from build123d import *

# Parameters (mm, degrees)
F1_DEPTH = 63.5
F2_DEPTH = 25.4
F0_W     = 25.3307413936
F0_H     = 19.05
F3_DEPTH = 50.8


with BuildPart() as f1:
    # F0 (on Front) → F1 (new body, symmetric)
    with BuildSketch(Plane.XZ):
        Polygon((-41.275, -9.525), (41.275, -9.525), (41.275, 9.525), (22.225, 9.525), (-41.275, 9.525), align=None)
    extrude(amount=F1_DEPTH, both=True)

    # F0 (on Front) → F2 (join, symmetric)
    with BuildSketch(Plane.XZ):
        with BuildLine():
            add(Edge.make_bspline(
                [(-41.275, 9.525), (-41.1319843278, 26.4440384857), (9.9134722481, 58.1405185942), (52.9354553425, 61.6699741315)],
                knots=[0, 0, 0, 0, 107.9558196003, 107.9558196003, 107.9558196003, 107.9558196003], degree=3))
            Line((-41.275, 9.525), (22.225, 9.525))
            Line((22.225, 9.525), (22.225, 27.0002))
            ThreePointArc((22.225, 27.0002), (31.0066586187, 50.1579487338), (52.9354553425, 61.6699741315))
        make_face()
    extrude(amount=F2_DEPTH, both=True)

    # F0 (on Front) → F3 (join, symmetric)
    with BuildSketch(Plane.XZ):
        with BuildLine():
            Line((22.225, 9.525), (41.275, 9.525))
            Line((41.275, 9.525), (41.275, 27.0002))
            ThreePointArc((41.275, 27.0002), (45.9246798487, 38.2255201513), (57.15, 42.8752))
            Line((57.15, 42.8752), (60.325, 42.8752))
            Line((60.325, 42.8752), (60.325, 61.9252))
            Line((60.325, 61.9252), (57.15, 61.9252))
            add(Edge.make_bspline(
                [(52.9354553425, 61.6699741315), (54.3496711259, 61.7859941605), (55.7552170324, 61.8715779158), (57.15, 61.9252)],
                knots=[107.9558196003, 107.9558196003, 107.9558196003, 107.9558196003, 111.5045361635, 111.5045361635, 111.5045361635, 111.5045361635], degree=3))
            ThreePointArc((52.9354553425, 61.6699741315), (31.0066586187, 50.1579487338), (22.225, 27.0002))
            Line((22.225, 27.0002), (22.225, 9.525))
        make_face()
        with Locations((72.9903706968, 52.4002)):
            Rectangle(F0_W, F0_H)
        Polygon((85.6557413936, 42.8752), (60.325, 42.8752), (60.325, 38.1), (111.125, 38.1), (111.125, 66.675), (60.325, 66.675), (60.325, 61.9252), (85.6557413936, 61.9252), align=None)
    extrude(amount=F3_DEPTH, both=True)


solid = f1.part
The listing builds one solid part. Answer for the finished solid, in the listing's coordinates (mm). A direction names the side the tool comes from. Coordinates: 2 decimals unless noted, no trailing zeros. Loops run counter-clockwise (first coordinate to the right, second up) from the corner with the lowest first, then second, coordinate; pieces in that order, holes last.
1) Find the intervals of material crossed by L1, parallel to Y at x = 42, z = 51.5; L2, parallel to X at y = 39, z = 1.5 (3 decimals); L3, parallel to Y at x = 4, z = 37.5, in increasing order.
2) Find section A-A on z = -2. Write down the section's boundary in (x, y) (3 decimals).
3) Flat-ended cylindrical pins translate along their axes: pin 1 Ø2 at (x, y) = (91.5, 16.5) entering from -Z; pin 2 Ø10 at (x, y) = (49, 24) entering from -Z; pin 3 Ø3.5 at (x, y) = (58.5, -13.5) entering from +Z; pin 4 Ø1 at (x, z) = (72, 37) entering from -Y. Find the tip coordinate at first contact, or state that the pin passes through.
4) Find section B-B on x = 75. Write down the section's boundary in (y, z) (3 decimals), then the cut area to 3 significant figures.
5) A tool of negligible diameter and unlimited length cuts with its end or side. For faces 1 (the face through (66, 50.8, 45)), 2 (the face through (85, -1, 38.1)), 3 (the face through (-4, 25.4, 30)), from which of +Z, -Z, +X, -X, +Y, -Y can it reach the whole face along a straight path? Write none if from no direction.
Values:
1. L1: y = -50.8 to 50.8
1. L2: x = -41.275 to 41.275
1. L3: y = -25.4 to 25.4
2. outline: (-41.275, -63.5) - (41.275, -63.5) - (41.275, 63.5) - (-41.275, 63.5) - close
3. pin 1: stops at z = 38.1
3. pin 2: stops at z = 35.89
3. pin 3: stops at z = 61.93
3. pin 4: passes through
4. outline: (-50.8, 38.1) - (50.8, 38.1) - (50.8, 66.675) - (-50.8, 66.675) - close
4. area: 2,900 mm2
5. face 1: +Z, +X, -X, +Y
5. face 2: -Z, +X, +Y, -Y
5. face 3: +Z, -X, +Y
